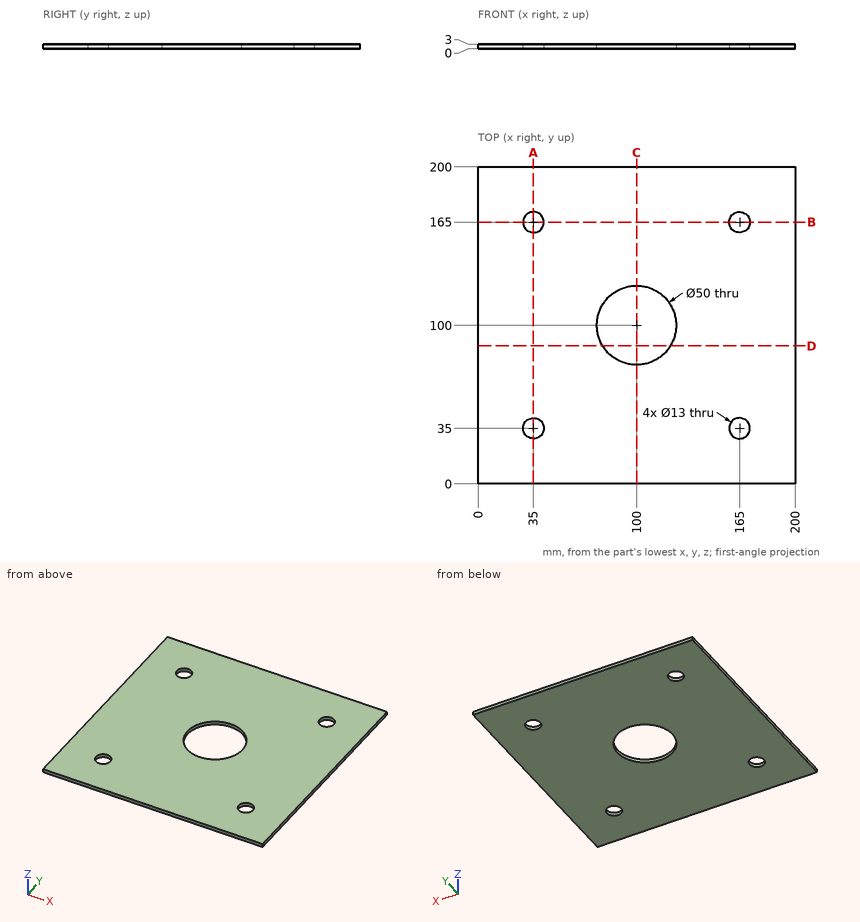
The drawing under review shows one solid part. Ordinate dimensions are in mm from its lowest x, y, z. Round coordinates to 2 decimals unless told otherwise and drop trailing zeros. Write each loop counter-clockwise with the first axis right and the second up, starting at its lowest first coordinate (ties: lowest second). Pieces come first, ordered by that corner, then holes. Notation, with made-up numbers: (55, -2) - (85, -2) arc R30 ccw to (85, 29) - close; hole circle Ø4 at (-21, -9.75). An arc over 180 degrees is marked (long way). Write each question's results on one line, items separated by ' | '.
Item 1: Take a section at A-A on x = 35. State the section outline as (y, z) points.
Calculated:
outline: (0, 0) - (28.5, 0) - (28.5, 3) - (0, 3) - close; (41.5, 0) - (158.5, 0) - (158.5, 3) - (41.5, 3) - close; (171.5, 0) - (200, 0) - (200, 3) - (171.5, 3) - close
Item 2: To check wall thickness, follow line 1 along X through (y, z) = (35, 1.55); line 2 along Y through (x, z) = (100, 0.8). State the ranges of each line that lie inside material, in increasing order. Write a range as from..to.
Calculated:
line 1: x = 0..28.5, 41.5..158.5, 171.5..200 | line 2: y = 0..75, 125..200
Item 3: Take a section at D-D on y = 87. State the section outline as (x, z) points.
Calculated:
outline: (0, 0) - (78.65, 0) - (78.65, 3) - (0, 3) - close; (121.35, 0) - (200, 0) - (200, 3) - (121.35, 3) - close
Item 4: Take a section at C-C on x = 100. State the section outline as (y, z) points.
Calculated:
outline: (0, 0) - (75, 0) - (75, 3) - (0, 3) - close; (125, 0) - (200, 0) - (200, 3) - (125, 3) - close
